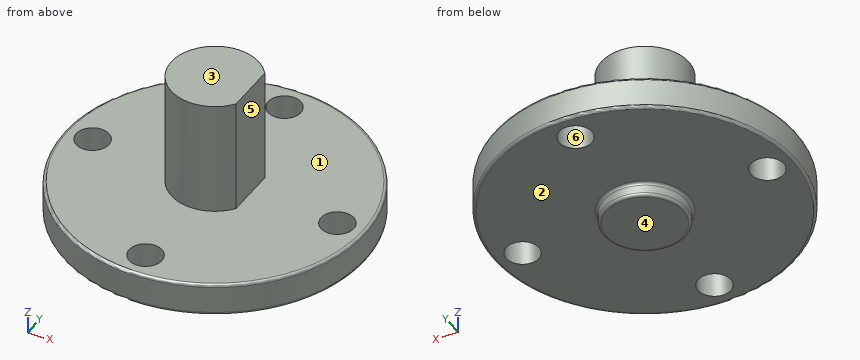
from build123d import *

# Parameters (mm, degrees)
F3_D     = 6
F4_R     = 0.5
F6_W     = 9.32738
F6_H     = 21
F7_DEPTH = 25


with BuildPart() as f1:
    # F0 (on Front) → F1 (revolve)
    with BuildSketch(Plane.XZ):
        Polygon((-7.5, -2.5), (0, -2.5), (0, 27), (-8, 27), (-8, 6), (-27.5, 6), (-27.5, 0), (-7.5, 0), align=None)
    revolve(axis=Axis((0, 0, 5.601703), (0, 0, -1)))

    # F3 (through all)
    with Locations(Plane(origin=(0, 0, 0), x_dir=(1, 0, 0), z_dir=(0, 0, -1))):
        with Locations((0, -22.5), (22.5, 0), (0, 22.5), (-22.5, 0)):
            Hole(F3_D / 2)

    # F4
    f4_edges = [f1.edges().sort_by_distance(p)[0] for p in [
        (27.5, 0, 6),
        (27.5, 0, 0),
        (7.5, 0, -2.5),
        (7.5, 0, 0),
    ]]
    fillet(f4_edges, radius=F4_R)

    # F6 (on offset) → F7 (cut)
    with BuildSketch(Plane.YZ.offset(6.5)):
        with Locations((0, 16.5)):
            Rectangle(F6_W, F6_H)
    extrude(amount=F7_DEPTH, mode=Mode.SUBTRACT)


solid = f1.part
Could you check a few things on this model? Use its own coordinates, in mm. Face numbers are marked on the shaded views. A direction names the side the tool comes from. Give positions to 0.01 mm unless a question says otherwise; leave off trailing zeros. Order: outer loops, then holes, each group sorted by start corner. A loop starts at its lowest first (then second) coordinate and runs counter-clockwise, first axis right, second up.
1. Suppose I cut it at D-D (z = 16). Write out the boundary of the cut face in (x, y).
Answers below:
outline: (6.5, -4.66) - (6.5, 4.66) arc R8 ccw (long way) to start
2. Which directions (+Z, -Z, +X, -X, +Y, -Y) give clear straight access to the entire face, cutting with the end or side of a thin tool? Please do the marked faces 1, 2 and 3.
Answers below:
face 1: +Z
face 2: -Z
face 3: +Z, +X, -X, +Y, -Y
3. For pin 1 (10 mm diameter, centred on y = 8.5, z = 7.5, fed in from +X); pin 2 (2 mm diameter, centred on x = -11.5, y = -12.5, fed in from -Z); pin 3 (2 mm diameter, centred on x = 14.5, y = 6.5, fed in from +Z); pin 4 (8 mm diameter, centred on x = 9.5, y = 5.5, fed in from +Z), each with a flat end and sliding along its axis, tell me the tip position at first contact or that it passes through.
Answers below:
pin 1: stops at x = 27.22
pin 2: stops at z = 0
pin 3: stops at z = 6
pin 4: stops at z = 27
4. Suppose I cut it at C-C (z = 1.75). Write out the boundary of the cut face in (x, y), plus the area to 3 significant figures.
Answers below:
outline: circle Ø55 at (0, 0); hole circle Ø6 at (-22.5, 0); hole circle Ø6 at (0, -22.5); hole circle Ø6 at (0, 22.5); hole circle Ø6 at (22.5, 0)
area: 2,260 mm2
5. Suppose I cut it at B-B (y = 0). Write out the boundary of the cut face in (x, z).
Answers below:
outline: (-27.5, 0.5) arc R0.5 ccw to (-27, 0) - (-25.5, 0) - (-25.5, 6) - (-27, 6) arc R0.5 ccw to (-27.5, 5.5) - close; (-19.5, 0) - (-8, 0) arc R0.5 cw to (-7.5, -0.5) - (-7.5, -2) arc R0.5 ccw to (-7, -2.5) - (7, -2.5) arc R0.5 ccw to (7.5, -2) - (7.5, -0.5) arc R0.5 cw to (8, 0) - (19.5, 0) - (19.5, 6) - (6.5, 6) - (6.5, 27) - (-8, 27) - (-8, 6) - (-19.5, 6) - close; (25.5, 0) - (27, 0) arc R0.5 ccw to (27.5, 0.5) - (27.5, 5.5) arc R0.5 ccw to (27, 6) - (25.5, 6) - close
6. Thinking about a two-plate mould opening in X: for the marked faces 4, 5 and 6, which applies, +X half, -X half, draft (parallel to the pull), parting line (faces both ways), or undercut?
Answers below:
face 4: draft
face 5: +X half
face 6: undercut
7. I need wall thicknesses on L1, parallel to Z at x = -8, y = -19; L2, parallel to X at y = -22.5, z = 3.5. Which ranges of each line are inside material? Lowest first, please.
Answers below:
L1: z = 0 to 6
L2: x = -15.81 to -3, 3 to 15.81
8. Suppose I cut it at A-A (x = 0). Write out the boundary of the cut face in (y, z).
Answers below:
outline: (-27.5, 0.5) arc R0.5 ccw to (-27, 0) - (-25.5, 0) - (-25.5, 6) - (-27, 6) arc R0.5 ccw to (-27.5, 5.5) - close; (-19.5, 0) - (-8, 0) arc R0.5 cw to (-7.5, -0.5) - (-7.5, -2) arc R0.5 ccw to (-7, -2.5) - (7, -2.5) arc R0.5 ccw to (7.5, -2) - (7.5, -0.5) arc R0.5 cw to (8, 0) - (19.5, 0) - (19.5, 6) - (8, 6) - (8, 27) - (-8, 27) - (-8, 6) - (-19.5, 6) - close; (25.5, 0) - (27, 0) arc R0.5 ccw to (27.5, 0.5) - (27.5, 5.5) arc R0.5 ccw to (27, 6) - (25.5, 6) - close
